Answer from the drawing. Dimensions are ordinates in mm from the lowest x, y and z of the part. A direction names the side the tool comes from. Give positions to 0.01 mm unless a question says otherwise; leave off trailing zeros. Write each loop counter-clockwise with the first axis right and the second up, starting at its lowest first coordinate (ties: lowest second). Pieces come first, ordered by that corner, then holes. Notation, with made-up numbers: (13, -22) -> (26, -22) arc R19 cw to (26, -3) -> close; hole circle Ø6 at (25, 79). An arc over 180 degrees is marked (long way). Put each result on its own line as item: value. Start each with the question number.
1) A cutting plane is placed at A-A (x = 17). Write down the section's boundary in (y, z) (1 decimal), then the cut area to 3 significant figures.
2) Flat-ended cylindrical pins translate along their axes: pin 1 Ø6.5 at (x, y) = (45.5, 12) entering from -Z; pin 2 Ø6.5 at (y, z) = (14.5, 39.5) entering from -X; pin 3 Ø14 at (y, z) = (8, 38) entering from +X (1 decimal). Find the tip coordinate at first contact, or state that the pin passes through.
3) A cutting plane is placed at D-D (x = 44). Write down the section's boundary in (y, z).
4) Find the intervals of material crossed by line 1 along X through (y, z) = (16.25, 72) (1 decimal); line 2 along Z through (x, y) = (80, 21.5); line 3 along Z through (x, y) = (78.5, 5.25) (1 decimal), in increasing order. Write a range as from..to.
5) For the marked faces 1, 2, 3, 4 and 5, determine the directions among +Z, -Z, +X, -X, +Y, -Y from which every point of the face is accessible in a straight line to the end or side of a thin tool.
6) A cutting plane is placed at C-C (z = 5). Write down the section's boundary in (x, y) (1 decimal), then the cut area to 3 significant figures.
7) For a pull along Z with two mould halves and no side action, classify the marked faces 6, 7, 8 and 9 as released by +Z, released by -Z, zero draft, split by the parting line, or undercut.
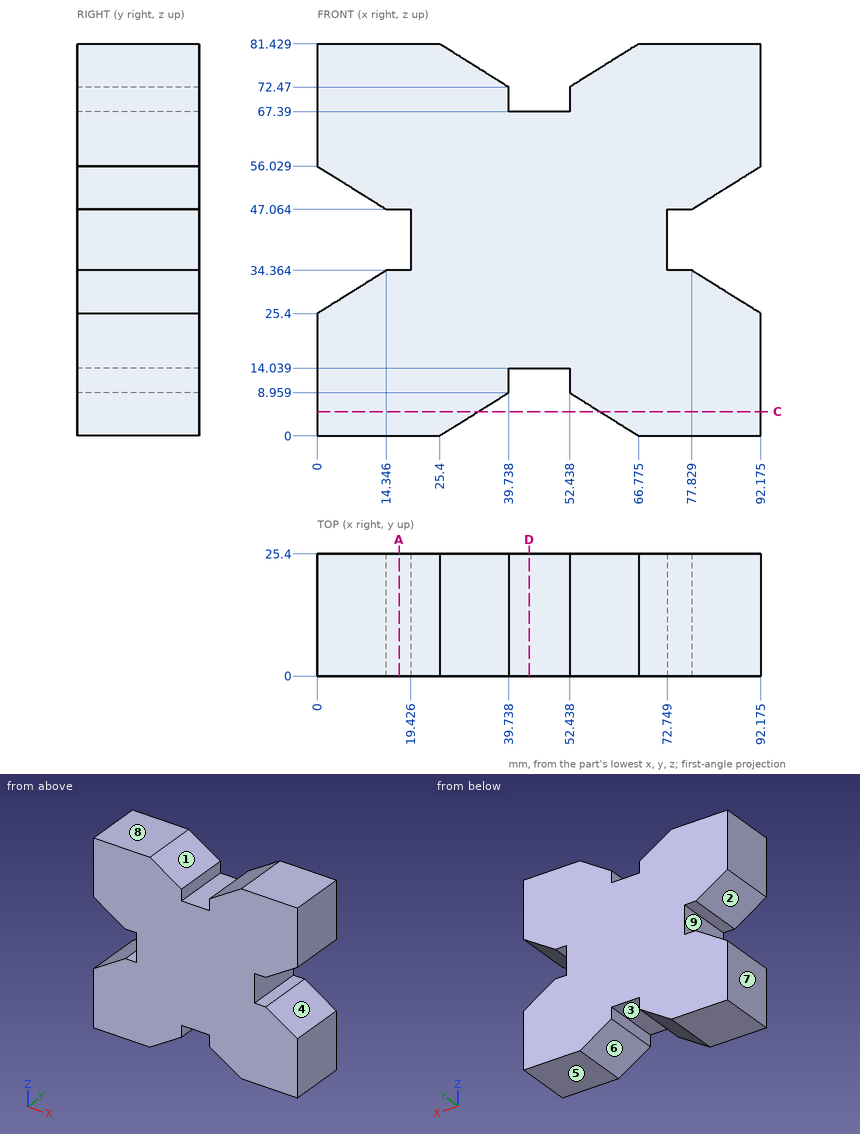
Reply:
1. outline: (0, 0) -> (25.4, 0) -> (25.4, 34.4) -> (0, 34.4) -> close; (0, 47.1) -> (25.4, 47.1) -> (25.4, 81.4) -> (0, 81.4) -> close
1. area: 1,750 mm2
2. pin 1: stops at z = 14.04
2. pin 2: stops at x = 19.43
2. pin 3: stops at x = 83.2
3. outline: (0, 14.04) -> (25.4, 14.04) -> (25.4, 67.39) -> (0, 67.39) -> close
4. line 1: x = 0..39.7, 52.4..92.2
4. line 2: z = 0..33.01, 48.42..81.43
4. line 3: z = 0..33.9, 47.5..81.4
5. face 1: +Z, +Y, -Y
5. face 2: -X, +Y, -Y
5. face 3: -Z, +Y, -Y
5. face 4: +X, +Y, -Y
5. face 5: -Z, +X, -X, +Y, -Y
6. outline: (0, 0) -> (33.4, 0) -> (33.4, 25.4) -> (0, 25.4) -> close; (58.8, 0) -> (92.2, 0) -> (92.2, 25.4) -> (58.8, 25.4) -> close
6. area: 1,700 mm2
7. face 6: released by -Z
7. face 7: zero draft
7. face 8: released by +Z
7. face 9: undercut
